Design review of the part built by this model. Coordinates are the model's own, in mm. A direction names the side the tool comes from. Coordinates: 2 decimals unless noted, no trailing zeros. Loops run counter-clockwise (first coordinate to the right, second up) from the corner with the lowest first, then second, coordinate; pieces in that order, holes last. Notation, with made-up numbers: (24.25, -1) - (43.25, -1) arc R13 cw to (43.25, 10) - close; hole circle Ø3 at (17.25, 4). An arc over 180 degrees is marked (long way). Return JSON: item names as keys, results as strings. Group by question number.
from build123d import *

# Parameters (mm, degrees)
SKETCH_1_W               = 210
SKETCH_1_H               = 200
EXTRUDE_1_DEPTH          = 3
CUT_EXTRUDE_1_DEPTH      = 291.015516826
FILLET_2_R               = 10
FILLET_3_R               = 5
CUT_EXTRUDE_2_DEPTH      = 291.015516826
CUT_EXTRUDE_2_DEPTH_BACK = 291.015516826
SKETCH_4_R               = 1.5
SKETCH_5_R               = 1.5
CUT_EXTRUDE_3_DEPTH      = 291.015516826


with BuildPart() as part:
    # 草图1 → 凸台-拉伸1 (new body)
    with BuildSketch(Plane.XY):
        with Locations((105, 100)):
            Rectangle(SKETCH_1_W, SKETCH_1_H)
    extrude(amount=EXTRUDE_1_DEPTH)

    # 草图2 → 切除-拉伸1 (cut, through all)
    with BuildSketch(Plane.XY.offset(3)):
        with BuildLine():
            Line((43, 180), (43, 30))
            ThreePointArc((43, 30), (35, 22), (27, 30))
            Line((27, 30), (27, 180))
            ThreePointArc((27, 180), (35, 188), (43, 180))
        make_face()
        with BuildLine():
            Line((167, 180), (167, 30))
            ThreePointArc((167, 30), (175, 22), (183, 30))
            Line((183, 30), (183, 180))
            ThreePointArc((183, 180), (175, 188), (167, 180))
        make_face()
        with BuildLine():
            Line((93, 180), (93, 30))
            ThreePointArc((93, 30), (85, 22), (77, 30))
            Line((77, 30), (77, 180))
            ThreePointArc((77, 180), (85, 188), (93, 180))
        make_face()
        with BuildLine():
            Line((117, 180), (117, 30))
            ThreePointArc((117, 30), (125, 22), (133, 30))
            Line((133, 30), (133, 180))
            ThreePointArc((133, 180), (125, 188), (117, 180))
        make_face()
    extrude(amount=-CUT_EXTRUDE_1_DEPTH, mode=Mode.SUBTRACT)

    # 圆角2
    fillet_2_edges = [part.edges().sort_by_distance(p)[0] for p in [
        (210, 0, 1.5),
        (0, 0, 1.5),
    ]]
    fillet(fillet_2_edges, radius=FILLET_2_R)

    # 圆角3
    fillet_3_edges = [part.edges().sort_by_distance(p)[0] for p in [
        (0, 200, 1.5),
        (210, 200, 1.5),
    ]]
    fillet(fillet_3_edges, radius=FILLET_3_R)

    # 草图4 → 切除-拉伸2 (cut, two sides: drawn at the far end of the back side and taken through both)
    with BuildSketch(Plane.XY.offset(3).offset(-CUT_EXTRUDE_2_DEPTH_BACK)):
        with Locations((12.5, 3.5)):
            Circle(SKETCH_4_R)
        with Locations((37.5, 3.5)):
            Circle(SKETCH_4_R)
        with Locations(Location((172.5, 3.5, 0), (0, 0, 180))):
            Circle(SKETCH_4_R)
        with Locations(Location((197.5, 3.5, 0), (0, 0, 180))):
            Circle(SKETCH_4_R)
    extrude(amount=CUT_EXTRUDE_2_DEPTH + CUT_EXTRUDE_2_DEPTH_BACK, mode=Mode.SUBTRACT)

    # 草图5 → 切除-拉伸3 (cut, through all)
    with BuildSketch(Plane.XY.offset(3)):
        with Locations((97, 48)):
            Circle(SKETCH_5_R)
        with Locations((97, 30)):
            Circle(SKETCH_5_R)
        with Locations((97, 73)):
            Circle(SKETCH_5_R)
        with Locations((97, 91)):
            Circle(SKETCH_5_R)
    extrude(amount=-CUT_EXTRUDE_3_DEPTH, mode=Mode.SUBTRACT)


solid = part.part
Item 1: Add section D-D (x = 176.5). State the section outline as (y, z) points, then the cut area to 3 significant figures.
Item 2: Add section C-C (z = 1.5). Give the number of separate pieces and of enclosed holes in the cut face, then the cut area to 3 significant figures.
Item 3: Add section B-B (y = 135.5). State the section outline as (x, z) points.
Item 4: To check wall thickness, follow line 1 (X direction, y = 109.5, z = 0.2); line 2 (X direction, y = 91, z = 1.3); line 3 (Y direction, x = 97, z = 1.1). State the ranges of each line that lie inside material, in increasing order. Write a range as from..to.
Item 5: For faces 1 (the face through (85, 22, 2)), 2 (the face through (104, 101, 3)), list the 3-axis set-ups (+Z, -Z, +X, -X, +Y, -Y) from which the entire face can be reached by the end or side of a thin tool; tool diameter is ignored.
Item 6: Draft analysis for pull direction X (two halves, no side actions). For faces 3 (the face through (35, 188, 2)), 4 (the face through (208, 199, 2)), 5 (the face through (2.85, 3.01, 1.52)), state which applies: pulls with the +X half, pulls with the -X half, needs draft (parallel to the pull), parting line crosses it, or undercut.
Item 7: For P1, Ø2.5, axis at x = 97, y = 30, coming from the +Z side, flat-tipped, find the tip position at first contact; note if it passes through.
Item 8: Add section A-A (x = 85). State the section outline as (y, z) points, then the cut area to 3 significant figures.
Answers below:
{
 "1": {"outline": "(0, 0) - (22.14, 0) - (22.14, 3) - (0, 3) - close; (187.86, 0) - (200, 0) - (200, 3) - (187.86, 3) - close", "area": "103 mm^2"},
 "2": {"separate pieces": "1", "enclosed holes": "12", "area": "31,500 mm^2"},
 "3": {"outline": "(0, 0) - (27, 0) - (27, 3) - (0, 3) - close; (43, 0) - (77, 0) - (77, 3) - (43, 3) - close; (93, 0) - (117, 0) - (117, 3) - (93, 3) - close; (133, 0) - (167, 0) - (167, 3) - (133, 3) - close; (183, 0) - (210, 0) - (210, 3) - (183, 3) - close"},
 "4": {"line 1": "x = 0..27, 43..77, 93..117, 133..167, 183..210", "line 2": "x = 0..27, 43..77, 93..95.5, 98.5..117, 133..167, 183..210", "line 3": "y = 0..28.5, 31.5..46.5, 49.5..71.5, 74.5..89.5, 92.5..200"},
 "5": {"face 1": "+Z, -Z", "face 2": "+Z, +X, -X, +Y, -Y"},
 "6": {"face 3": "undercut", "face 4": "pulls with the +X half", "face 5": "pulls with the -X half"},
 "7": {"P1": "passes through"},
 "8": {"outline": "(0, 0) - (22, 0) - (22, 3) - (0, 3) - close; (188, 0) - (200, 0) - (200, 3) - (188, 3) - close", "area": "102 mm^2"}
}
